from build123d import *

# Parameters (mm, degrees)
SKETCH1_R           = 1.6
BOSS_EXTRUDE1_DEPTH = 1
THICKEN2_START      = -5.917392258
THICKEN2_DEPTH      = 11.834784516


# Read off the part's stored shape, not the designer's step: Thicken2
with BuildPart() as part:
    # Sketch1 → Boss-Extrude1 (new body)
    with BuildSketch(Plane(origin=(0, 0, 0), x_dir=(1, 0, 0), z_dir=(0, 1, 0))):
        with BuildLine():
            Line((-11.1, 4.202456856), (-11.1, -3.525300194))
            ThreePointArc((-11.1, -3.525300194), (-9.45, -5.175300194), (-7.8, -3.525300194))
            ThreePointArc((-7.8, -3.525300194), (-7.04227284, -2.555092036), (-5.917392258, -3.055190021))
            Line((-5.917392258, -3.055190021), (5.917392258, -3.055190021))
            ThreePointArc((5.917392258, -3.055190021), (7.04227284, -2.555092036), (7.8, -3.525300194))
            ThreePointArc((7.8, -3.525300194), (9.45, -5.175300194), (11.1, -3.525300194))
            Line((11.1, -3.525300194), (11.1, 4.202456856))
            add(Edge.make_bspline(
                [(11.1, 4.202456856), (5.688924475, 8.144809979), (0, 8.144809979)],
                knots=[0, 0, 0, 1, 1, 1], degree=2))
            add(Edge.make_bspline(
                [(-11.1, 4.202456856), (-5.688924475, 8.144809979), (0, 8.144809979)],
                knots=[0, 0, 0, 1, 1, 1], degree=2))
        make_face()
        with Locations(Location((-6.8, 0, 0), (0, 0, 270))):
            Circle(SKETCH1_R, mode=Mode.SUBTRACT)
        with Locations(Location((6.8, 0, 0), (0, 0, 90))):
            Circle(SKETCH1_R, mode=Mode.SUBTRACT)
    extrude(amount=BOSS_EXTRUDE1_DEPTH)

    # Thicken2 outline → Thicken2 (add)
    with BuildSketch(Plane.YZ.offset(THICKEN2_START)):
        with BuildLine():
            Line((2.877817459, 3.833007481), (4.098758354, 2.612066586))
            Line((4.098758354, 2.612066586), (4.805865135, 3.319173367))
            Line((4.805865135, 3.319173367), (3.58492424, 4.540114262))
            ThreePointArc((3.58492424, 4.540114262), (1.296364791, 4.99533704), (0, 3.055190021))
            Line((0, 3.055190021), (1, 3.055190021))
            ThreePointArc((1, 3.055190021), (1.679048224, 4.071457507), (2.877817459, 3.833007481))
        make_face()
    extrude(amount=THICKEN2_DEPTH)


solid = part.part
The listing builds one solid part. Answer for the finished solid, in the listing's coordinates (mm). A direction names the side the tool comes from. Coordinates: 2 decimals unless noted, no trailing zeros. Loops run counter-clockwise (first coordinate to the right, second up) from the corner with the lowest first, then second, coordinate; pieces in that order, holes last. Notation, with made-up numbers: M 67.5,-34 L 122.5,-34 A30 cw 122.5,-1 Z; hole C 39,7.5 d3. An arc over 180 degrees is marked long. Answer in a Markdown table with one row per item.
1) Which of the six approach directions +Z, -Z, +X, -X, +Y, -Y give full straight-line access (tool end or side, diameter ignored) to faces 5 (the flat face through (-0.08, 3.48, 3.23)), 6 (the cylindrical face through (-0.08, 1.33, 5.01)), 7 (the flat face through (-11.1, 0.5, -0.4))?
Answers below:
| item | result |
|---|---|
| face 5 | -Z, +X, -X |
| face 6 | +Z |
| face 7 | +Z, -Z, -X, +Y, -Y |
2) Determine the mould class of faces 1 (the cylindrical face through (5.214, 0.493, 0.208)), 2 (the cylindrical face through (-7.06, 0.49, 2.56)), 3 (the flat face through (11.1, 0.5, -0.3)), 4 (the cylindrical face through (-0.083, 1.662, 4.064)) for opening direction Z: released by +Z, released by -Z, zero draft, split by the parting line, or undercut.
Answers below:
| item | result |
|---|---|
| face 1 | undercut |
| face 2 | released by +Z |
| face 3 | zero draft |
| face 4 | released by -Z |
3) Find the intervals of material crossed by probe 1 along X at (y, z) = (0.9, 0); probe 2 along Y at (x, z) = (-4.25, 3); probe 3 along Z at (x, y) = (6.8, 0.5), in increasing order.
Answers below:
| item | result |
|---|---|
| probe 1 | -11.1 to -8.4, -5.2 to 5.2, 8.4 to 11.1 |
| probe 2 | 0 to 1, 3.71 to 4.49 |
| probe 3 | -6.69 to -1.6, 1.6 to 2.53 |
4) Find section A-A (z = 0). Determine the outline of the cut face in (x, y).
Answers below:
| item | result |
|---|---|
| outline | M -11.1,0 L -8.4,0 L -8.4,1 L -11.1,1 Z; M -5.2,0 L 5.2,0 L 5.2,1 L -5.2,1 Z; M 8.4,0 L 11.1,0 L 11.1,1 L 8.4,1 Z |
5) Find section B-B (y = 4.4). Determine the outline of the cut face in (x, z).
Answers below:
| item | result |
|---|---|
| outline | M -5.92,2.91 L 5.92,2.91 L 5.92,3.73 L -5.92,3.73 Z |
6) Given pin 1 (2 mm diameter, centred on x = 2, z = 1, fed in from +Y); pin 2 (2.5 mm diameter, centred on x = 6.8, z = 0, fed in from +Y), each flat-ended and moving along its own axis, determine where each tip first touches the part or whether it passes through.
Answers below:
| item | result |
|---|---|
| pin 1 | y = 1 |
| pin 2 | through |
